Could you check a few things on this model? Use its own coordinates, in mm. Face numbers are marked on the shaded views. A direction names the side the tool comes from. Give positions to 0.01 mm unless a question says otherwise; leave off trailing zeros. Write each loop counter-clockwise with the first axis right and the second up, starting at its lowest first coordinate (ties: lowest second). Pieces come first, ordered by that corner, then holes. Notation, with made-up numbers: (-10, 33) - (28, 33) arc R34 cw to (28, 71) - close; hole circle Ø4 at (-7, -18.75). An arc over 180 degrees is marked (long way). Use one line per item in the form item = value.
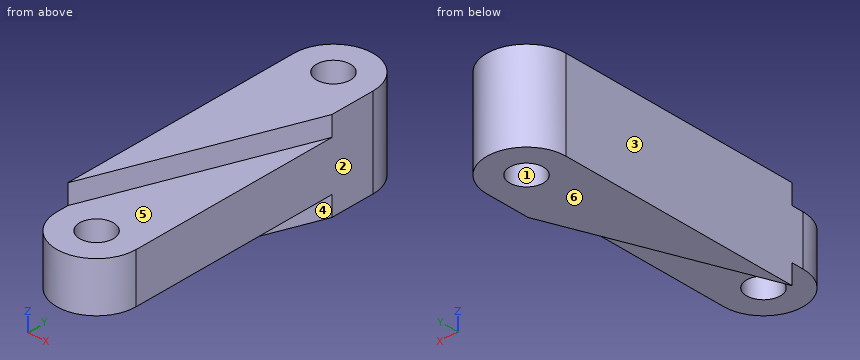
Autodesk Inventor part; units mm, degrees
ref_plane "YZ Plane" through (0, 0, 0) normal (1, 0, 0) x (0, 1, 0)
ref_plane "XZ Plane" through (0, 0, 0) normal (0, 1, 0) x (-1, 0, 0)
ref_plane "XY Plane" through (0, 0, 0) normal (0, 0, 1) x (1, 0, 0)
sketch "Sketch1" plane through (0, 0, 0) normal (0, 0, 1) x (1, 0, 0)
  line L0 (0, 17.1345) -> (0, 17.1345)
  line L1 (4, 13.1345) -> (4, 8.5672)
  line L2 (0, -17.1345) -> (0, -17.1345)
  line L3 (-4, -13.1345) -> (-4, -11.9123)
  line L4 (-4, 17.1345) -> (0, 17.1345) construction
  line L5 (0, 17.1345) -> (0, 0) construction
  line L6 (0, 0) -> (-4, 0) construction
  line L7 (-4, 0) -> (-4, 17.1345) construction
  arc A0 (4, 13.1345) -> (0, 17.1345) centre (0, 13.1345) ccw
  arc A1 (0, 17.1345) -> (-4, 13.1345) centre (0, 13.1345) ccw
  arc A2 (-4, -13.1345) -> (0, -17.1345) centre (0, -13.1345) ccw
  arc A3 (0, -17.1345) -> (4, -13.1345) centre (0, -13.1345) ccw
  line L8 (-4, -11.9123) -> (4, 8.5672)
  line L9 (4, 8.5672) -> (4, -13.1345)
  line L10 (-4, -11.9123) -> (-4, 13.1345)
  dimension "d0" = 4
  dimension "d6" = 26.269
extrude "Extrusion1" add sketch "Sketch1" along normal mid plane 9 contours L1 L8 L10 A1 A0
extrude "Extrusion2" add sketch "Sketch1" along normal mid plane 5 contours L9 A3 A2 L3 L8
sketch "Sketch2" plane through (0, 0, 4.5) normal (0, 0, 1) x (1, 0, 0)
  arc A0 (4, 13.1345) -> (-4, 13.1345) centre (0, 13.1345) ccw construction
  line L0 (-4, -13.1345) -> (-4, -11.9123)
  arc A1 (-4, -13.1345) -> (4, -13.1345) centre (0, -13.1345) ccw
  line L1 (4, 8.5672) -> (4, -13.1345)
  line L2 (-4, -11.9123) -> (4, 8.5672)
  point P0 (0, 0)
hole "Hole1" at (0, 13.1345, 4.5) at (0, -13.1345, 4.5) direction (0, 0, -1) diameter 3.4 end through all
equation "\"d6\" = LengthC"
properties part number "F"
1. Imagine slicing it at A-A, the plane x = -1. List the corners of the cut face in (y, z) for me.
Response values:
outline = (-17.01, -2.5) - (-14.51, -2.5) - (-14.51, 2.5) - (-17.01, 2.5) - close; (-11.76, -2.5) - (-4.23, -2.5) - (-4.23, -4.5) - (11.76, -4.5) - (11.76, 4.5) - (-4.23, 4.5) - (-4.23, 2.5) - (-11.76, 2.5) - close; (14.51, -4.5) - (17.01, -4.5) - (17.01, 4.5) - (14.51, 4.5) - close
2. If we mould it in two halves opening along X, with no side actions, what happens to the marked faces 1, 2 and 3? For each: pulls with the +X half, pulls with the -X half, needs draft (parallel to the pull), parting line crosses it, or undercut.
Response values:
face_1 = undercut
face_2 = pulls with the +X half
face_3 = pulls with the -X half
3. For pin 1 (1.5 mm diameter, centred on x = -0.5, y = -8, fed in from -Z); pin 2 (1.5 mm diameter, centred on x = -1.5, z = 2, fed in from -Y), each with a flat end and sliding along its axis, tell me the tip position at first contact or that it passes through.
Response values:
pin_1 = -2.5
pin_2 = -17.06
4. Which directions (+Z, -Z, +X, -X, +Y, -Y) give clear straight access to the entire face, cutting with the end or side of a thin tool? Please do the marked faces 4, 5 and 6.
Response values:
face_4 = -Z, +X, -Y
face_5 = +Z, +X, -Y
face_6 = -Z, +X, -X, +Y, -Y
5. Imagine slicing it at B-B, the plane z = -0.75. List the corners of the cut face in (x, y) for me.
Response values:
outline = (-4, -13.13) arc R4 ccw to (4, -13.13) - (4, 13.13) arc R4 ccw to (-4, 13.13) - close; hole circle Ø3.4 at (0, -13.13); hole circle Ø3.4 at (0, 13.13)
6. Imagine slicing it at C-C, the plane y = -5.5. List the corners of the cut face in (x, z) for me.
Response values:
outline = (-4, -4.5) - (-1.5, -4.5) - (-1.5, -2.5) - (4, -2.5) - (4, 2.5) - (-1.5, 2.5) - (-1.5, 4.5) - (-4, 4.5) - close
7. Imagine slicing it at D-D, the plane x = 3. List the corners of the cut face in (y, z) for me.
Response values:
outline = (-15.78, -2.5) - (6.01, -2.5) - (6.01, -4.5) - (15.78, -4.5) - (15.78, 4.5) - (6.01, 4.5) - (6.01, 2.5) - (-15.78, 2.5) - close
8. If I drill on line 1 (Y direction, x = 0, z = -1.75); line 2 (Z direction, x = 2.75, y = -14.5); line 3 (Y direction, x = 0.25, z = 2), over which ranges is the centre line in solid material (lowest first)? Write a range as from..to.
Response values:
line_1 = -17.13..-14.83, -11.43..11.43, 14.83..17.13
line_2 = -2.5..2.5
line_3 = -17.13..-14.82, -11.45..11.45, 14.82..17.13
